Autodesk Inventor part; units mm, degrees
ref_plane "YZ Plane" through (0, 0, 0) normal (1, 0, 0) x (0, 1, 0)
ref_plane "XZ Plane" through (0, 0, 0) normal (0, 1, 0) x (-1, 0, 0)
ref_plane "XY Plane" through (0, 0, 0) normal (0, 0, 1) x (1, 0, 0)
sketch "Sketch1" plane through (0, 0, 0) normal (0, 0, 1) x (1, 0, 0)
  circle A0 centre (0, 0) radius 3.175
  circle A1 centre (0, 0) radius 5
  circle A2 centre (0, 0) radius 11
  circle A3 centre (0, 8) radius 1.5
  circle A4 centre (-8, 0) radius 1.5
  circle A5 centre (0, -8) radius 1.5
  circle A6 centre (8, 0) radius 1.5
  dimension "d0" = 22
  dimension "d1" = 6.35
  dimension "d2" = 10
  dimension "d3" = 3
  dimension "d4" = 8
  dimension "d7" = 360
extrude "Extrusion1" add sketch "Sketch1" along normal blind 12 contours A1
extrude "Extrusion2" add sketch "Sketch1" along normal blind 2 contours A2
chamfer "Chamfer1" distance 0.5 angle 45 2 edges at (-5, 0, 2) (-5, 0, 12)
sketch "Sketch3" plane through (0, 0, 0) normal (0, 1, 0) x (-1, 0, 0)
  circle A0 centre (0, 7.5211) radius 1.5
  point P0 (0, 0)
  dimension "d16" = 3
extrude "Extrusion3" cut sketch "Sketch3" against normal blind 10
equation "\"BendRadius\" = Thickness"
equation "\"BendReliefWidth\" = Thickness"
equation "\"BendReliefDepth\" = 0.5 * Thickness"
equation "\"CornerReliefSize\" = 4 * Thickness"
equation "\"MinimumRemnant\" = 2 * Thickness"
equation "\"TransitionRadius\" = BendRadius"
equation "\"JacobiRadiusSize\" = BendRadius"
equation "\"GapSize\" = Thickness"
properties part number "mặt bích"
Geometry: final body of the model. Coordinates: model frame, mm. A direction names the side the tool comes from. Coordinates: 2 decimals unless noted, no trailing zeros. Order: outer loops, then holes, each group sorted by start corner. A loop starts at its lowest first (then second) coordinate and runs counter-clockwise, first axis right, second up. Notation, with made-up numbers: (34.5, 3) - (91.5, 3) arc R23 cw to (91.5, 16) - close; hole circle Ø4 at (42, 3). An arc over 180 degrees is marked (long way). Return JSON: item names as keys, results as strings. Group by question number.
1. Cut plane A-A (x = 0). Output: boundary loops of the cut face in (y, z) (3 decimals), plus the area to 3 significant figures.
2. Cut plane B-B (y = 0). Output: boundary loops of the cut face in (x, z) (3 decimals), plus the area to 3 significant figures.
3. Material intervals for line 1 along Z through (x, y) = (-8.5, 3.25); line 2 along Y through (x, z) = (-8, 0.9); line 3 along X through (y, z) = (-2, 10.75), sorted ascending. Write a range as [from, to].
4. Set-up query: faces 4 (the face through (-1.43, -3.88, 7.97)), 5 (the face through (2, 3, 0)), 6 (the face through (-1.08, 4.88, 6.94)). Return all of +Z, -Z, +X, -X, +Y, -Y with unobstructed straight access to the full face (end or side cutting, diameter ignored); none if empty.
5. Cut plane C-C (z = 1.5). Output: boundary loops of the cut face in (x, y) (3 decimals).
6. Cut plane D-D (y = -8). Output: boundary loops of the cut face in (x, z).
7. Pin query (flat end, axial travel): pin 1 (4 mm diameter, centred on x = 0, y = 0, fed in from -Z); pin 2 (1 mm diameter, centred on x = 8, y = -3.5, fed in from +Z); pin 3 (3.5 mm diameter, centred on x = 0, z = 7.52, fed in from -Y); pin 4 (2 mm diameter, centred on y = -2.5, z = 6.5, fed in from -X). Return the tip coordinate at first contact, or that it passes through.
8. Pull-direction query (X, two-part tool) for faces 1 (the face through (-9.5, -0.07, 0.99)), 2 (the face through (-2.38, 10.74, 0.99)), 3 (the face through (-3, 5, 2)); classes: pulls with the +X half, pulls with the -X half, needs draft (parallel to the pull), parting line crosses it, or undercut.
Resolved:
{
 "1": {"outline": "(-11, 0) - (-9.5, 0) - (-9.5, 2) - (-11, 2) - close; (-6.5, 0) - (-3.175, 0) - (-3.175, 6.021) - (-5, 6.021) - (-5, 2.5) - (-5.5, 2) - (-6.5, 2) - close; (-5, 9.021) - (-3.175, 9.021) - (-3.175, 12) - (-4.5, 12) - (-5, 11.5) - close; (3.175, 0) - (6.5, 0) - (6.5, 2) - (5.5, 2) - (5, 2.5) - (5, 11.5) - (4.5, 12) - (3.175, 12) - close; (9.5, 0) - (11, 0) - (11, 2) - (9.5, 2) - close", "area": "50.3 mm²"},
 "2": {"outline": "(-11, 0) - (-9.5, 0) - (-9.5, 2) - (-11, 2) - close; (-6.5, 0) - (-3.175, 0) - (-3.175, 12) - (-4.5, 12) - (-5, 11.5) - (-5, 2.5) - (-5.5, 2) - (-6.5, 2) - close; (3.175, 0) - (6.5, 0) - (6.5, 2) - (5.5, 2) - (5, 2.5) - (5, 11.5) - (4.5, 12) - (3.175, 12) - close; (9.5, 0) - (11, 0) - (11, 2) - (9.5, 2) - close", "area": "55.8 mm²"},
 "3": {"line 1": "z = [0, 2]", "line 2": "y = [-7.55, -1.5], [1.5, 7.55]", "line 3": "x = [-4.58, -2.47], [2.47, 4.58]"},
 "4": {"face 4": "-Y", "face 5": "-Z, +X, -X, +Y, -Y", "face 6": "+Z"},
 "5": {"outline": "circle Ø22 at (0, 0); hole circle Ø3 at (-8, 0); hole circle Ø6.35 at (0, 0); hole circle Ø3 at (0, -8); hole circle Ø3 at (0, 8); hole circle Ø3 at (8, 0)"},
 "6": {"outline": "(-7.55, 0) - (-1.5, 0) - (-1.5, 2) - (-7.55, 2) - close; (1.5, 0) - (7.55, 0) - (7.55, 2) - (1.5, 2) - close"},
 "7": {"pin 1": "passes through", "pin 2": "stops at z = 2", "pin 3": "stops at y = -5", "pin 4": "stops at x = -4.77"},
 "8": {"face 1": "undercut", "face 2": "parting line crosses it", "face 3": "needs draft"}
}
